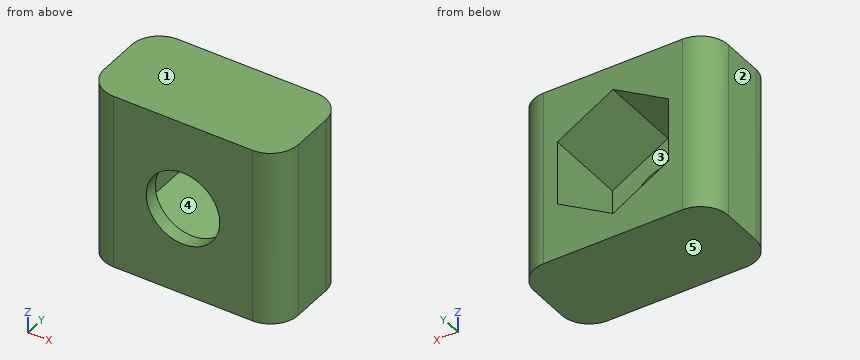
```python
from build123d import *

# Parameters (mm, degrees)
SKETCH1_W            = 14
SKETCH1_H            = 7
BOSS_EXTRUDE1_DEPTH  = 6.35
CUT_EXTRUDE1_DEPTH   = 6
FILLET1_R            = 2
M5_CLEARANCE_HOLE1_D = 5.3


with BuildPart() as part:
    # Sketch1 → Boss-Extrude1 (new, symmetric)
    with BuildSketch(Plane.XY):
        with Locations((0, -3.5)):
            Rectangle(SKETCH1_W, SKETCH1_H)
    extrude(amount=BOSS_EXTRUDE1_DEPTH, both=True)

    # Sketch2 → Cut-Extrude1 (cut)
    with BuildSketch(Plane(origin=(0, 0, 0), x_dir=(1, 0, 0), z_dir=(0, 1, 0))):
        Polygon((0, -4.618802154), (4, -2.309401077), (4, 2.309401077), (0, 4.618802154), (-4, 2.309401077), (-4, -2.309401077), align=None)
    extrude(amount=-CUT_EXTRUDE1_DEPTH, mode=Mode.SUBTRACT)

    # Fillet1
    fillet1_edges = [part.edges().sort_by_distance(p)[0] for p in [
        (7, -7, 0),
        (-7, -7, 0),
        (-7, 0, 0),
        (7, 0, 0),
    ]]
    fillet(fillet1_edges, radius=FILLET1_R)

    # M5 Clearance Hole1 (through all)
    with Locations(Plane(origin=(0, -7, 0), x_dir=(-1, 0, 0), z_dir=(0, -1, 0))):
        with Locations((0, 0)):
            Hole(M5_CLEARANCE_HOLE1_D / 2)


solid = part.part
```
Part model, mm, in its own coordinate system. Face numbers are marked on the shaded views. A direction names the side the tool comes from. Give positions to 0.01 mm unless a question says otherwise; leave off trailing zeros. Order: outer loops, then holes, each group sorted by start corner. A loop starts at its lowest first (then second) coordinate and runs counter-clockwise, first axis right, second up. Notation, with made-up numbers: (18, 30) - (36, 30) arc R17 cw to (36, 46) - close; hole circle Ø7 at (65.5, 81.25). An arc over 180 degrees is marked (long way). Use one line per item in the form item = value.
Item 1: Slice it at A-A on z = 0. Give the cut face in (x, y).
Solution:
outline = (-7, -5) arc R2 ccw to (-5, -7) - (-2.65, -7) - (-2.65, -6) - (-4, -6) - (-4, 0) - (-5, 0) arc R2 ccw to (-7, -2) - close; (2.65, -7) - (5, -7) arc R2 ccw to (7, -5) - (7, -2) arc R2 ccw to (5, 0) - (4, 0) - (4, -6) - (2.65, -6) - close
Item 2: Probe probe 1 along Z at (x, y) = (0, -6.75); probe 2 along X at (y, z) = (-4, 1); probe 3 along X at (y, z) = (-1.5, 1). List the from-to ranges inside material, lowest first. Write a range as from..to.
Solution:
probe_1 = -6.35..-2.65, 2.65..6.35
probe_2 = -7..-4, 4..7
probe_3 = -6.94..-4, 4..6.94
Item 3: Pin check, flat tip, straight feed: pin 1 Ø5 at (x, z) = (0, 0) entering from +Y. Stop position of the tip, or through.
Solution:
pin_1 = through
Item 4: Two-plate mould, pull along X, no slides. Class the marked faces 1, 2 and 3: released by +X, released by -X, zero draft, split by the parting line, or undercut.
Solution:
face_1 = zero draft
face_2 = released by -X
face_3 = undercut
Item 5: Slice it at B-B on y = -2.5. Give the cut face in (x, z), and give its area (3 significant figures).
Solution:
outline = (-7, -6.35) - (7, -6.35) - (7, 6.35) - (-7, 6.35) - close; hole (-4, -2.31) - (0, -4.62) - (4, -2.31) - (4, 2.31) - (0, 4.62) - (-4, 2.31) - close
area = 122 mm2
Item 6: Which spindle directions (+Z, -Z, +X, -X, +Y, -Y) get a long thin tool onto all of the face, cutting with end or side? Do the marked faces 4 and 5. Say none if no direction does.
Solution:
face_4 = +Y
face_5 = -Z, +X, -X, +Y, -Y
Item 7: Slice it at D-D on y = -5.25. Give the cut face in (x, z).
Solution:
outline = (-6.98, -6.35) - (6.98, -6.35) - (6.98, 6.35) - (-6.98, 6.35) - close; hole (-4, -2.31) - (0, -4.62) - (4, -2.31) - (4, 2.31) - (0, 4.62) - (-4, 2.31) - close
Item 8: Slice it at C-C on z = -4. Give the cut face in (x, y).
Solution:
outline = (-7, -5) arc R2 ccw to (-5, -7) - (5, -7) arc R2 ccw to (7, -5) - (7, -2) arc R2 ccw to (5, 0) - (1.07, 0) - (1.07, -6) - (-1.07, -6) - (-1.07, 0) - (-5, 0) arc R2 ccw to (-7, -2) - close
